Verification items for the finished model (mm, model axes). Give positions to 0.01 mm unless a question says otherwise; leave off trailing zeros. Loops run counter-clockwise (first coordinate to the right, second up) from the corner with the lowest first, then second, coordinate; pieces in that order, holes last. Notation, with made-up numbers: M 58.25,20 L 63.25,20 A31 ccw 63.25,46 Z; hole C 56,-4.75 d11. An arc over 180 degrees is marked long. Answer in a Markdown table with one row per item.
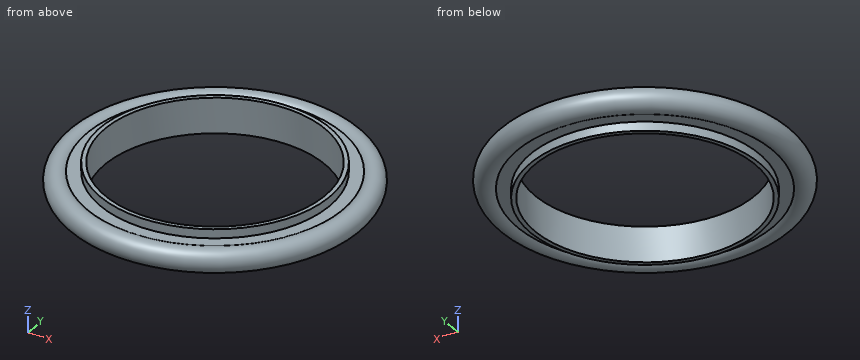
```python
from build123d import *


with BuildPart() as part:
    # Sketch1 → Revolve1 (revolve)
    with BuildSketch(Plane(origin=(0, 0, 0), x_dir=(0, 0, -1), z_dir=(1, 0, 0)), mode=Mode.PRIVATE) as revolve1_sk:
        with BuildLine():
            Line((-4, 25), (4, 25))
            Line((4, 25), (4, 26))
            Line((4, 26), (1.95, 26))
            Line((1.95, 26), (1.95, 28.94745668))
            ThreePointArc((1.95, 28.94745668), (0, 33.391892525), (-1.95, 28.94745668))
            Line((-1.95, 28.94745668), (-1.95, 26))
            Line((-1.95, 26), (-4, 26))
            Line((-4, 26), (-4, 25))
        make_face()
    revolve(revolve1_sk.sketch.rotate(Axis((0, 0, -6.803273839), (0, 0, -1)), 90), axis=Axis((0, 0, -6.803273839), (0, 0, -1)))


solid = part.part
```
Item 1: Go/stop test with flat-tipped pins: pin 1 (4 mm diameter, centred on x = -12, z = -1.5, fed in from -Y); pin 2 (4 mm diameter, centred on y = 4, z = 0.5, fed in from +X); pin 3 (3 mm diameter, centred on y = 23, z = 0, fed in from -X). Record where each tip stops, or that it passes through.
Reported:
| item | result |
|---|---|
| pin 1 | stops at y = -31.72 |
| pin 2 | stops at x = 33.33 |
| pin 3 | stops at x = -25.55 |
Item 2: Scan lines: L1, parallel to Y at x = 0, z = -2; L2, parallel to Y at x = 0, z = -1; L3, parallel to Y at x = 0, z = -0.5. Record each from-to range of solid material in increasing order. Write a range as [from, to].
Reported:
| item | result |
|---|---|
| L1 | y = [-32.48, -29], [-26, -25], [25, 26], [29, 32.48] |
| L2 | y = [-33.2, -25], [25, 33.2] |
| L3 | y = [-33.34, -25], [25, 33.34] |
Item 3: Sectioned sample at C-C (z = 1). Record the cut outline in (x, y).
Reported:
| item | result |
|---|---|
| outline | C 0,0 d66.39; hole C 0,0 d50 |
Item 4: Sectioned sample at A-A (y = 0). Record the cut outline in (x, z).
Reported:
| item | result |
|---|---|
| outline | M -28.95,-1.95 L -26,-1.95 L -26,-4 L -25,-4 L -25,4 L -26,4 L -26,1.95 L -28.95,1.95 A2.65 ccw long Z; M 25,-4 L 26,-4 L 26,-1.95 L 28.95,-1.95 A2.65 ccw long 28.95,1.95 L 26,1.95 L 26,4 L 25,4 Z |
